from build123d import *

# Parameters (mm, degrees)
SKETCH1_R           = 50.8
BOSS_EXTRUDE1_DEPTH = 6.35
SKETCH2_W           = 6.35
SKETCH2_H           = 67.818
BOSS_EXTRUDE2_DEPTH = 57.15
SKETCH3_W           = 2.54
SKETCH3_H           = 12.7
BOSS_EXTRUDE3_DEPTH = 12.500000082
SKETCH4_W           = 2
SKETCH4_H           = 12.7
BOSS_EXTRUDE4_DEPTH = 3
SKETCH5_W           = 2
SKETCH5_H           = 12.7
BOSS_EXTRUDE5_DEPTH = 2.5
SKETCH6_OUTSIDE_W   = 135.018
SKETCH6_OUTSIDE_H   = 135.018
SKETCH6_OUTSIDE_W_2 = 46.379926406
SKETCH6_OUTSIDE_H_2 = 67.818
CUT_EXTRUDE1_DEPTH  = 7.35


with BuildPart() as part:
    # Sketch1 → Boss-Extrude1 (new body)
    with BuildSketch(Plane(origin=(0, 0, 0), x_dir=(1, 0, 0), z_dir=(0, 1, 0))):
        Circle(SKETCH1_R)
    extrude(amount=BOSS_EXTRUDE1_DEPTH)

    # Sketch2 → Boss-Extrude2 (add)
    with BuildSketch(Plane(origin=(0, 6.35, 0), x_dir=(1, 0, 0), z_dir=(0, 1, 0))):
        with Locations((17.804926406, 0)):
            Rectangle(SKETCH2_W, SKETCH2_H)
    extrude(amount=BOSS_EXTRUDE2_DEPTH)

    # Sketch3 → Boss-Extrude3 (add)
    with BuildSketch(Plane(origin=(20.979926406, 0, 0), x_dir=(0, 0, -1), z_dir=(1, 0, 0))):
        with Locations((-32.52, 34.925)):
            Rectangle(SKETCH3_W, SKETCH3_H)
        with Locations((32.52, 34.925)):
            Rectangle(SKETCH3_W, SKETCH3_H)
    extrude(amount=BOSS_EXTRUDE3_DEPTH)

    # Sketch4 → Boss-Extrude4 (add)
    with BuildSketch(Plane(origin=(0, 0, 31.25), x_dir=(-1, 0, 0), z_dir=(0, 0, -1))):
        with Locations((-32.479926488, 34.925)):
            Rectangle(SKETCH4_W, SKETCH4_H)
    extrude(amount=BOSS_EXTRUDE4_DEPTH)

    # Sketch5 → Boss-Extrude5 (add)
    with BuildSketch(Plane.XY.offset(-31.25)):
        with Locations((32.479926488, 34.925)):
            Rectangle(SKETCH5_W, SKETCH5_H)
    extrude(amount=BOSS_EXTRUDE5_DEPTH)

    # Sketch6 outside → Cut-Extrude1 (cut, through all)
    with BuildSketch(Plane(origin=(0, 6.35, 0), x_dir=(1, 0, 0), z_dir=(0, 1, 0))):
        Rectangle(SKETCH6_OUTSIDE_W, SKETCH6_OUTSIDE_H)
        with Locations((-2.210036797, 0)):
            Rectangle(SKETCH6_OUTSIDE_W_2, SKETCH6_OUTSIDE_H_2, mode=Mode.SUBTRACT)
    extrude(amount=-CUT_EXTRUDE1_DEPTH, mode=Mode.SUBTRACT)


solid = part.part
Could you check a few things on this model? Use its own coordinates, in mm. A direction names the side the tool comes from. Give positions to 0.01 mm unless a question says otherwise; leave off trailing zeros. Order: outer loops, then holes, each group sorted by start corner. A loop starts at its lowest first (then second) coordinate and runs counter-clockwise, first axis right, second up.
1. Suppose I cut it at D-D (y = 48.5). List the corners of the cut face in (x, z) for me, plus the area to 3 significant figures.
2. Suppose I cut it at B-B (y = 31). List the corners of the cut face in (x, z) for me, plus the area to 3 significant figures.
3. Suppose I cut it at A-A (z = 11). List the corners of the cut face in (x, y) for me, plus the area to 3 significant figures.
4. We'd pull the mould along Z, two halves only. Please class faces 1 (the flat face through (32, 35, -28.75)), 2 (the flat face through (27, 35, -33.79)), 3 (the flat face through (26, 35, -31.25)), 4 (the flat face through (27, 41.275, -32)): pulls with the +Z half, pulls with the -Z half, needs draft (parallel to the pull), parting line crosses it, or undercut.
5. Will these pins go through, and if not, where does the flat tip stop? P1, Ø19, axis at y = 35, z = 14.5, coming from the +X side; P2, Ø6, axis at x = 26, z = 31.5, coming from the -Y side (3 decimals); P3, Ø0.9, axis at y = 34.5, z = 29.5, coming from the -X side; P4, Ø1.5, axis at x = 19.5, z = -16, coming from the -Y side.
6. Suppose I cut it at C-C (x = -20). List the corners of the cut face in (y, z) for me.
7. I need wall thicknesses on L1, parallel to Y at x = 7.5, z = -5.5; L2, parallel to X at y = 39.5, z = 2.5; L3, parallel to X at y = 5, z = 29. Which ranges of each line are inside material? Lowest first, please.
8. For faces 5 (the flat face through (27, 28.575, -32)), 6 (the flat face through (32, 35, 28.25)), 7 (the flat face through (29, 41.275, 32)), 8 (the flat face through (31.48, 35, -30)), which set-ups out of +Z, -Z, +X, -X, +Y, -Y let a thin tool reach every point of the face, with its end or its side?
Solved:
1. outline: (14.63, -33.91) - (20.98, -33.91) - (20.98, 33.91) - (14.63, 33.91) - close
1. area: 431 mm2
2. outline: (14.63, -33.91) - (20.98, -33.91) - (20.98, -33.79) - (33.48, -33.79) - (33.48, -28.75) - (31.48, -28.75) - (31.48, -31.25) - (20.98, -31.25) - (20.98, 31.25) - (31.48, 31.25) - (31.48, 28.25) - (33.48, 28.25) - (33.48, 33.79) - (20.98, 33.79) - (20.98, 33.91) - (14.63, 33.91) - close
2. area: 505 mm2
3. outline: (-25.4, 0) - (20.98, 0) - (20.98, 63.5) - (14.63, 63.5) - (14.63, 6.35) - (-25.4, 6.35) - close
3. area: 657 mm2
4. face 1: undercut
4. face 2: pulls with the -Z half
4. face 3: undercut
4. face 4: needs draft
5. P1: stops at x = 20.98
5. P2: stops at y = 28.575
5. P3: stops at x = 14.63
5. P4: stops at y = 0
6. outline: (0, -33.91) - (6.35, -33.91) - (6.35, 33.91) - (0, 33.91) - close
7. L1: y = 0 to 6.35
7. L2: x = 14.63 to 20.98
7. L3: x = -25.4 to 20.98
8. face 5: +Z, -Z, +X, -Y
8. face 6: +X, +Y, -Y
8. face 7: +Z, -Z, +X, +Y
8. face 8: +Y, -Y
